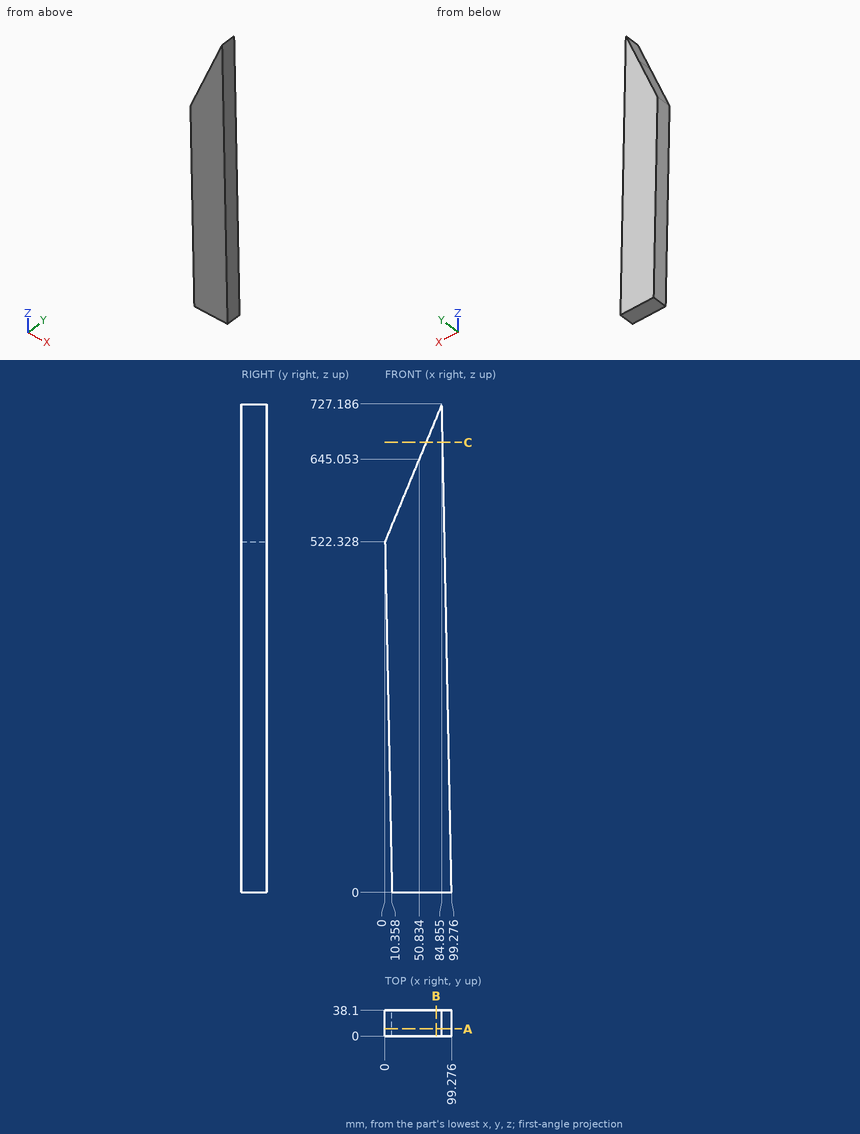
Answer from the drawing. Dimensions are ordinates in mm from the lowest x, y and z of the part. Coordinates: 2 decimals unless noted, no trailing zeros. Loops run counter-clockwise (first coordinate to the right, second up) from the corner with the lowest first, then second, coordinate; pieces in that order, holes last. Notation, with made-up numbers: (45, -33.5) -> (71, -33.5) arc R34 cw to (71, 2.5) -> close; hole circle Ø8 at (-4.75, 8.25). An arc over 180 degrees is marked (long way). Answer in a Markdown table with one row per item.
Item 1: A cutting plane is placed at B-B on x = 76. Determine the outline of the cut face in (y, z).
Returned:
| item | result |
|---|---|
| outline | (0, 0) -> (38.1, 0) -> (38.1, 705.81) -> (0, 705.81) -> close |
Item 2: Straight lines are drawn through the part: line 1 along Z through (x, y) = (62.5, 25) (1 decimal); line 2 along X through (y, z) = (26, 144.5); line 3 along X through (y, z) = (6.5, 632.5) (1 decimal). For each, find the intervals that lie inside material, in ascending order. Write a range as [from, to].
Returned:
| item | result |
|---|---|
| line 1 | z = [0, 673.2] |
| line 2 | x = [7.49, 96.41] |
| line 3 | x = [45.6, 86.7] |
Item 3: A cutting plane is placed at A-A on y = 10.5. Determine the outline of the cut face in (x, z) (1 decimal).
Returned:
| item | result |
|---|---|
| outline | (0, 522.3) -> (10.4, 0) -> (99.3, 0) -> (84.9, 727.2) -> (50.8, 645.1) -> close |
Item 4: A cutting plane is placed at C-C on z = 670. Determine the outline of the cut face in (x, y), plus the area to 3 significant figures.
Returned:
| item | result |
|---|---|
| outline | (61.17, 0) -> (85.99, 0) -> (85.99, 38.1) -> (61.17, 38.1) -> close |
| area | 946 mm^2 |
Item 5: Each of these flat-tipped pins is pushed along its axis until it touches: P1, Ø6, axis at x = 51, y = 29, coming from the +Z side (1 decimal); P2, Ø4, axis at x = 40.5, y = 26.5, coming from the +Z side (1 decimal); P3, Ø12, axis at y = 5, z = 641.5, coming from the -X side; P4, Ø1.5, axis at x = 37.5, z = 333, coming from the -Y side. Where does it stop, or does it pass through?
Returned:
| item | result |
|---|---|
| P1 | stops at z = 652.7 |
| P2 | stops at z = 624.9 |
| P3 | stops at x = 46.88 |
| P4 | stops at y = 0 |
